Check sheet for the modelled part. Datum: model origin and axes. Units: mm. A direction names the side the tool comes from. Round coordinates to 2 decimals unless told otherwise and drop trailing zeros. Order: outer loops, then holes, each group sorted by start corner. A loop starts at its lowest first (then second) coordinate and runs counter-clockwise, first axis right, second up.
```python
from build123d import *

# Parameters (mm, degrees)
SKETCH1_R           = 10
SKETCH1_R_2         = 1.5
BOSS_EXTRUDE1_DEPTH = 2
SKETCH2_R           = 4.5
SKETCH2_R_2         = 3
BOSS_EXTRUDE2_DEPTH = 3
SKETCH3_R           = 1
CUT_EXTRUDE1_DEPTH  = 2
CIRPATTERN1_COUNT   = 4


with BuildPart() as part:
    # Sketch1 → Boss-Extrude1 (new body)
    with BuildSketch(Plane.XY):
        Circle(SKETCH1_R)
        Circle(SKETCH1_R_2, mode=Mode.SUBTRACT)
    extrude(amount=BOSS_EXTRUDE1_DEPTH)

    # Sketch2 → Boss-Extrude2 (add)
    with BuildSketch(Plane.XY.offset(2)):
        Circle(SKETCH2_R)
        Circle(SKETCH2_R_2, mode=Mode.SUBTRACT)
    extrude(amount=BOSS_EXTRUDE2_DEPTH)

    # Sketch3 → Cut-Extrude1 (cut)
    with BuildSketch(Plane(origin=(0, 0, 0), x_dir=(-1, 0, 0), z_dir=(0, 0, -1))):
        with Locations((0, 7)):
            Circle(SKETCH3_R)
    cut_extrude1 = extrude(amount=-CUT_EXTRUDE1_DEPTH, mode=Mode.SUBTRACT)

    # CirPattern1: Cut-Extrude1 ×4 about axis
    cirpattern1_axis = Axis((0, 0, 0), (0, 0, 1))
    for i in range(1, CIRPATTERN1_COUNT):
        add(cut_extrude1.rotate(cirpattern1_axis, i * 360 / CIRPATTERN1_COUNT), mode=Mode.SUBTRACT)


solid = part.part
```
Item 1: Go/stop test with flat-tipped pins: P1, Ø2.5, axis at x = 0, y = -7, coming from the +Z side; P2, Ø2, axis at y = 6.5, z = 1, coming from the +X side. Record where each tip stops, or that it passes through.
Answer:
P1: stops at z = 2
P2: stops at x = 8.35
Item 2: Sectioned sample at C-C (z = 1.25). Record the cut outline in (x, y).
Answer:
outline: circle Ø20 at (0, 0); hole circle Ø2 at (-7, 0); hole circle Ø3 at (0, 0); hole circle Ø2 at (0, -7); hole circle Ø2 at (0, 7); hole circle Ø2 at (7, 0)
Item 3: Sectioned sample at A-A (x = 0). Record the cut outline in (y, z).
Answer:
outline: (-10, 0) - (-8, 0) - (-8, 2) - (-10, 2) - close; (-6, 0) - (-1.5, 0) - (-1.5, 2) - (-3, 2) - (-3, 5) - (-4.5, 5) - (-4.5, 2) - (-6, 2) - close; (1.5, 0) - (6, 0) - (6, 2) - (4.5, 2) - (4.5, 5) - (3, 5) - (3, 2) - (1.5, 2) - close; (8, 0) - (10, 0) - (10, 2) - (8, 2) - close
Item 4: Release check for a two-part mould opening along X. For faces 1 (the cylindrical face through (8, 0, 1)), 2 (the flat face through (1, -3, 5)), 3 (the cylindrical face through (-0.59, 4.46, 3.48)) record: released by +X, released by -X, zero draft, split by the parting line, or undercut.
Answer:
face 1: undercut
face 2: zero draft
face 3: split by the parting line
Item 5: Sectioned sample at D-D (x = 7). Record the cut outline in (y, z).
Answer:
outline: (-7.14, 0) - (-1, 0) - (-1, 2) - (-7.14, 2) - close; (1, 0) - (7.14, 0) - (7.14, 2) - (1, 2) - close
Item 6: Scan lines: line 1 along Y through (x, z) = (0, 1.1); line 2 along Y through (x, z) = (0, 3.85); line 3 along Z through (x, y) = (0, -9). Record each from-to range of solid material in increasing order.
Answer:
line 1: y = -10 to -8, -6 to -1.5, 1.5 to 6, 8 to 10
line 2: y = -4.5 to -3, 3 to 4.5
line 3: z = 0 to 2
Item 7: Access from +Z, -Z, +X, -X, +Y, -Y to the whole of each face (thin tool, end or side, straight path). Record for faces 4 (the cylindrical face through (-8, 0, 1)), 5 (the flat face through (4.3, -2.1, 2)).
Answer:
face 4: +Z, -Z
face 5: +Z
Item 8: Sectioned sample at B-B (y = -0.75). Record the cut outline in (x, z), and give its area (3 significant figures).
Answer:
outline: (-9.97, 0) - (-7.66, 0) - (-7.66, 2) - (-9.97, 2) - close; (-6.34, 0) - (-1.3, 0) - (-1.3, 2) - (-2.9, 2) - (-2.9, 5) - (-4.44, 5) - (-4.44, 2) - (-6.34, 2) - close; (1.3, 0) - (6.34, 0) - (6.34, 2) - (4.44, 2) - (4.44, 5) - (2.9, 5) - (2.9, 2) - (1.3, 2) - close; (7.66, 0) - (9.97, 0) - (9.97, 2) - (7.66, 2) - close
area: 38.6 mm2
